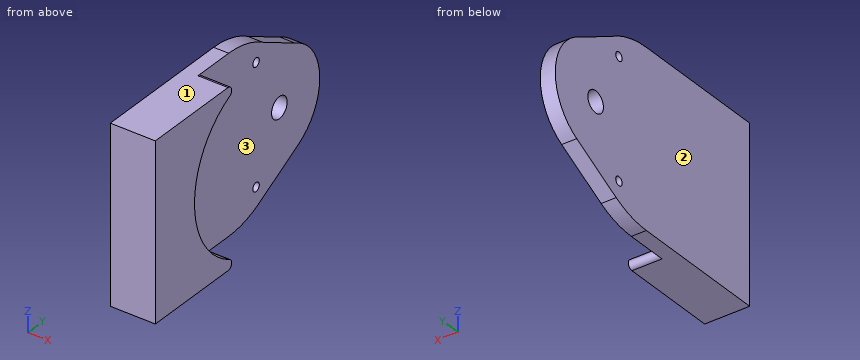
Autodesk Inventor part; units mm, degrees
ref_plane "YZ Plane" through (0, 0, 0) normal (1, 0, 0) x (0, 1, 0)
ref_plane "XZ Plane" through (0, 0, 0) normal (0, 1, 0) x (-1, 0, 0)
ref_plane "XY Plane" through (0, 0, 0) normal (0, 0, 1) x (1, 0, 0)
sketch "Sketch3" plane through (0, 0, 0) normal (1, 0, 0) x (0, 1, 0)
  line L0 (0, 0) -> (56.36, 0)
  line L1 (56.36, 70) -> (0, 70)
  line L2 (0, 70) -> (0, 0)
  circle A0 centre (84, 35) radius 4.25
  line L3 (84, 35) -> (56.36, 35)
  line L4 (96, 53.4391) -> (74.4743, 64.9114)
  line L5 (94.3473, 15.5852) -> (72.8216, 4.1129)
  arc A1 (94.3473, 15.5852) -> (92.6159, 55.2427) centre (84, 35) ccw
  arc A2 (74.9172, 64.6754) -> (56.36, 70) centre (56.36, 35) ccw
  arc A3 (56.36, 0) -> (72.8216, 4.1129) centre (56.36, 35) ccw
  line L6 (84, 35) -> (71.3, 35)
  line L7 (71.3, 35) -> (71.3, 58.82)
  line L8 (71.3, 58.82) -> (71.3, 35)
  line L9 (71.3, 35) -> (71.3, 11.18)
  circle A4 centre (71.3, 58.82) radius 1.75
  circle A5 centre (71.3, 11.18) radius 1.75
  dimension "d31" = 8.5
  dimension "d33" = 27.64
  dimension "d35" = 12.7
  dimension "d36" = 23.82
  dimension "d37" = 23.82
  dimension "d38" = 3.5
  dimension "d40" = 3.5
  dimension "d41" = 84
extrude "Extrusion3" add sketch "Sketch3" along normal blind 18
sketch "Sketch4" plane through (18, 0, 0) normal (1, 0, 0) x (0, 0, -1)
  line L0 (-35, 84) -> (-35, 56.36)
  arc A0 (-70, 56.36) -> (0, 56.36) centre (-35, 56.36) ccw
  line L1 (0, 56.36) -> (-35, 56.36)
  line L2 (-70, 56.36) -> (-70, 106)
  line L3 (-70, 106) -> (0, 106)
  line L4 (0, 106) -> (0, 56.36)
  point P0 (0, 0)
  dimension "d44" = 27.64
extrude "Extrusion4" cut sketch "Sketch4" against normal blind 12
fillet "Fillet1" radius 2 2 edges at (12, 56.36, 70) (12, 56.36, 0)
properties part number "Suporte Motor"
Build history of the part. All positions in model axes, mm. Face numbers are marked on the shaded views. Coordinates: 2 decimals unless noted, no trailing zeros. Order: outer loops, then holes, each group sorted by start corner. A loop starts at its lowest first (then second) coordinate and runs counter-clockwise, first axis right, second up.
Item 1: Drop flat-ended pins along their axis: pin 1 Ø3 at (x, z) = (15.5, 45) entering from +Y; pin 2 Ø2 at (y, z) = (71.3, 11.18) entering from -X; pin 3 Ø4 at (x, z) = (3.5, 48.5) entering from +Y (3 decimals); pin 4 Ø11 at (y, z) = (84, 35) entering from +X. Give the stop position or say it passes through.
Filled in:
pin 1: stops at y = 23.3
pin 2: passes through
pin 3: stops at y = 102.755
pin 4: stops at x = 6
Item 2: Saw through at D-D on y = 84. List the corners of the cut face in (x, z), then the cut area to 3 significant figures.
Filled in:
outline: (0, 10.07) - (6, 10.07) - (6, 30.75) - (0, 30.75) - close; (0, 39.25) - (6, 39.25) - (6, 59.83) - (0, 59.83) - close
area: 248 mm2
Item 3: Saw through at B-B on y = 71. List the corners of the cut face in (x, z), then the cut area to 3 significant figures.
Filled in:
outline: (0, 3.21) - (6, 3.21) - (6, 9.46) - (0, 9.46) - close; (0, 12.9) - (6, 12.9) - (6, 57.1) - (0, 57.1) - close; (0, 60.54) - (6, 60.54) - (6, 66.79) - (0, 66.79) - close
area: 340 mm2
Item 4: Mould opens along Z. For the marked faces 1, 2 and 3 say: released by +Z, released by -Z, zero draft, split by the parting line, or undercut.
Filled in:
face 1: released by +Z
face 2: zero draft
face 3: undercut
Item 5: Saw through at C-C on z = 11.18. List the corners of the cut face in (x, y).
Filled in:
outline: (0, 0) - (18, 0) - (18, 30.72) - (6, 30.72) - (6, 69.55) - (0, 69.55) - close; (0, 73.05) - (6, 73.05) - (6, 86.08) - (0, 86.08) - close
Item 6: Drill centre lines: L1, parallel to Z at x = 2.7, y = 71.3; L2, parallel to Y at x = 5.75, z = 59; L3, parallel to Y at x = 3.05, z = 11.18. Where is each one in solid material? Low to high.
Filled in:
L1: z = 3.35 to 9.43, 12.93 to 57.07, 60.57 to 66.65
L2: y = 0 to 69.56, 73.04 to 85.57
L3: y = 0 to 69.55, 73.05 to 86.08
Item 7: Saw through at A-A on x = 4. List the corners of the cut face in (y, z), then the cut area to 3 significant figures.
Filled in:
outline: (0, 0) - (56.36, 0) arc R35 ccw to (72.82, 4.11) - (94.35, 15.59) arc R22 ccw to (92.62, 55.24) - (74.92, 64.68) arc R35 ccw to (56.36, 70) - (0, 70) - close; hole circle Ø3.5 at (71.3, 11.18); hole circle Ø3.5 at (71.3, 58.82); hole circle Ø8.5 at (84, 35)
area: 6,380 mm2
